from build123d import *

# Parameters (mm, degrees)
SKETCH1_R           = 7.999999999999998
SKETCH1_R_2         = 7
BOSS_EXTRUDE1_DEPTH = 5
FILLET1_R           = 1
BOSS_EXTRUDE2_DEPTH = 0.85
SKETCH4_R           = 2
CUT_EXTRUDE1_DEPTH  = 16.23285921946369
FILLET3_R           = 1
FILLET4_R           = 1


# Some blends are built 0.0001 mm under size
with BuildPart() as part:
    # Sketch1 → Boss-Extrude1 (new, symmetric)
    with BuildSketch(Plane.XY):
        Circle(SKETCH1_R)
        Circle(SKETCH1_R_2, mode=Mode.SUBTRACT)
    extrude(amount=BOSS_EXTRUDE1_DEPTH, both=True)

    # Fillet1
    fillet1_edges = [part.edges().sort_by_distance(p)[0] for p in [
        (-7.999999999999998, 9.8e-16, -5),
        (-7.999999999999998, 9.8e-16, 5),
    ]]
    fillet(fillet1_edges, radius=FILLET1_R - 0.0001)  # a hair under: the kernel refuses the full size

    # Sketch2 → Revolve1 (revolve)
    with BuildSketch(Plane(origin=(0, 0, 0), x_dir=(1, 0, 0), z_dir=(0, 1, 0))):
        Polygon((4e-17, 5), (1.26e-15, -5), (-2.099999999999999, -4.999999999999999), (-2.0999999999999996, -5.200000000000002), (-2.6999999999999993, -5.200000000000002), (-3.4670223660818085, -0.8500000000000001), (-5.503508426201579, -0.8500000000000006), (-6.199999999999999, -4.800000000000001), (-6.999999999999999, -4.800000000000001), (-7, 4.799999999999999), (-6.2, 4.799999999999999), (-5.503508426201579, 0.8499999999999993), (-3.4670223660818085, 0.8499999999999992), (-2.7000000000000006, 5.200000000000002), (-2.1000000000000005, 5.200000000000002), (-2.1, 4.999999999999999), align=None)
    revolve(axis=Axis((4e-17, 0, -5), (1.2e-16, 0, 1)))

    # Sketch3 → Boss-Extrude2 (add, symmetric)
    with BuildSketch(Plane(origin=(0, 0, 0), x_dir=(1, 0, 0), z_dir=(0, 1, 0))):
        Polygon((-2.546735183281943, 2.550000000000001), (-2.546735183281943, 0.8500000000000001), (-4.546735183281943, 0.850000000000001), (-4.546735183281943, 1.15), (-2.846735183281943, 2.5500000000000003), align=None)
    extrude(amount=BOSS_EXTRUDE2_DEPTH, both=True)

    # Sketch4 → Cut-Extrude1 (cut, through all)
    with BuildSketch(Plane(origin=(-6.1e-16, 0, -4.999999999999999), x_dir=(-1, 0, 0), z_dir=(0, 0, -1))):
        Circle(SKETCH4_R)
    extrude(amount=-CUT_EXTRUDE1_DEPTH, mode=Mode.SUBTRACT)

    # Fillet3
    # the kernel refuses this fillet: 1 mm, written as the material it takes off along each edge
    with BuildSketch(Plane(origin=(1.29e-15, 0, 5.200000000000003), x_dir=(-1, 0, 0), z_dir=(0, 1, 0))) as fillet3_piece_1:
        with BuildLine():
            CenterArc((1.8555509868612252, -0.9696621473355957), FILLET3_R, 9.99999999999983, 65.85072553441276)
            Line((2.100000000000001, 0), (2.1048889802627766, 0.01939324294671163))
            ThreePointArc((2.1048889802627766, 0.01939324294671163), (2.4000000000000004, 0.01999999999999957), (2.7000000000000006, 0.01999999999999957))
            Line((2.7000000000000006, 0.01999999999999957), (2.719696155060245, 0.00347296355333881))
            Line((2.719696155060245, 0.00347296355333881), (2.860054894933678, -0.7925410061153295))
            Line((2.860054894933678, -0.7925410061153295), (2.840358739873434, -0.7960139696686683))
        make_face()
    revolve(axis=Axis((1.29e-15, 0, 5.200000000000003), (1.2e-16, 0, 1)), mode=Mode.SUBTRACT)

    # Fillet4
    # the kernel refuses this fillet: 1 mm, written as the material it takes off along each edge
    with BuildSketch(Plane(origin=(1e-17, 0, -5.200000000000002), x_dir=(-1, 0, 0), z_dir=(0, 1, 0))) as fillet4_piece_1:
        with BuildLine():
            CenterArc((1.8555509868612252, 0.9696621473355957), FILLET4_R, 284.1492744655874, 65.85072553441279)
            Line((2.1000000000000005, 0), (2.104888980262776, -0.01939324294671163))
            ThreePointArc((2.104888980262776, -0.01939324294671163), (2.4000000000000004, -0.01999999999999957), (2.7000000000000006, -0.01999999999999957))
            Line((2.7000000000000006, -0.01999999999999957), (2.719696155060245, -0.00347296355333881))
            Line((2.719696155060245, -0.00347296355333881), (2.860054894933678, 0.7925410061153295))
            Line((2.860054894933678, 0.7925410061153295), (2.840358739873434, 0.7960139696686683))
        make_face()
    revolve(axis=Axis((1e-17, 0, -5.200000000000002), (1.2e-16, 0, 1)), mode=Mode.SUBTRACT)


solid = part.part
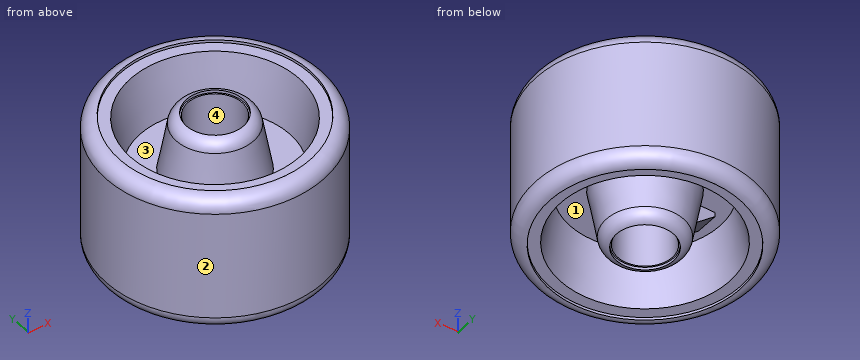
The listing builds one solid part. Answer for the finished solid, in the listing's coordinates (mm). Face numbers are marked on the shaded views. A direction names the side the tool comes from. Give positions to 0.01 mm unless a question says otherwise; leave off trailing zeros. Loops run counter-clockwise (first coordinate to the right, second up) from the corner with the lowest first, then second, coordinate; pieces in that order, holes last.
Item 1: Find the intervals of material crossed by line 1 along X through (y, z) = (-1.25, -3.5); line 2 along X through (y, z) = (2.5, 4.5); line 3 along X through (y, z) = (-1.5, 2.75), in increasing order.
Derived:
line 1: x = -7.9 to -5.84, -2.73 to -1.56, 1.56 to 2.73, 5.84 to 7.9
line 2: x = -7.46 to -5.62, -1.3 to 1.3, 5.62 to 7.46
line 3: x = -7.86 to -5.64, -2.75 to -1.32, 1.32 to 2.75, 5.64 to 7.86
Item 2: Each of these flat-tipped pins is pushed along its axis until it touches: pin 1 Ø6 at (x, y) = (4, -4.5) entering from +Z; pin 2 Ø1 at (x, z) = (-2, -0.5) entering from +Y; pin 3 Ø1 at (x, y) = (4.5, 1) entering from +Z. Where does it stop, or does it pass through?
Derived:
pin 1: stops at z = 5
pin 2: stops at y = 7.86
pin 3: stops at z = 0.85
Item 3: A cutting plane is placed at A-A (z = -2.75). Give the vertices of the cut face in (x, y).
Derived:
outline: circle Ø16 at (0, 0); circle Ø6.26 at (0, 0); hole circle Ø11.68 at (0, 0); hole circle Ø4 at (0, 0)
Item 4: Determine the mould class of the marked faces 1 and 2 for opening direction X: +X half, -X half, draft (parallel to the pull), parting line (faces both ways), or undercut.
Derived:
face 1: undercut
face 2: parting line
Item 5: A tool of negligible diameter and unlimited length cuts with its end or side. For the marked faces 3 and 4, from which of +Z, -Z, +X, -X, +Y, -Y can it reach the whole face along a straight path? Write none if from no direction.
Derived:
face 3: +Z
face 4: +Z, -Z
Item 6: A cutting plane is placed at B-B (z = 0.5). Give the vertices of the cut face in (x, y).
Derived:
outline: circle Ø16 at (0, 0); hole circle Ø4 at (0, 0)
